Read the model definition and answer for the solid it produces. Units are mm, in the model's axes. A direction names the side the tool comes from. Give positions to 0.01 mm unless a question says otherwise; leave off trailing zeros. Order: outer loops, then holes, each group sorted by start corner. A loop starts at its lowest first (then second) coordinate and runs counter-clockwise, first axis right, second up. Notation, with made-up numbers: M 88,74 L 146,74 A29 ccw 146,100 Z; hole C 22.25,69.25 d5. An arc over 180 degrees is marked long. One line per item, written item: value.
from build123d import *

# Parameters (mm, degrees)
SKETCH1_W          = 50
SKETCH1_H          = 50
SKETCH1_R          = 7.875
BASE_FLANGE1_DEPTH = 1
FILLET1_R          = 3
FILLET2_R          = 1
FILLET3_R          = 2


# Sheet-metal steps are written as plain solids
with BuildPart() as part:
    # Sketch1 → Base-Flange1 (new body)
    with BuildSketch(Plane(origin=(0, 0, 0), x_dir=(1, 0, 0), z_dir=(0, 1, 0))):
        Rectangle(SKETCH1_W, SKETCH1_H)
        with Locations(Location((0, 0, 0), (0, 0, 270))):
            Circle(SKETCH1_R, mode=Mode.SUBTRACT)
        with BuildLine():
            Line((20, 17.878679656), (20, -17.878679656))
            Line((20, -17.878679656), (7.962313054, -5.84099271))
            ThreePointArc((7.962313054, -5.84099271), (9.875, 0), (7.962313054, 5.84099271))
            Line((7.962313054, 5.84099271), (20, 17.878679656))
        make_face(mode=Mode.SUBTRACT)
        with BuildLine():
            Line((17.878679656, -20), (-17.878679656, -20))
            Line((-17.878679656, -20), (-5.84099271, -7.962313054))
            ThreePointArc((-5.84099271, -7.962313054), (0, -9.875), (5.84099271, -7.962313054))
            Line((5.84099271, -7.962313054), (17.878679656, -20))
        make_face(mode=Mode.SUBTRACT)
        with BuildLine():
            Line((-20, -17.878679656), (-20, 17.878679656))
            Line((-20, 17.878679656), (-7.962313054, 5.84099271))
            ThreePointArc((-7.962313054, 5.84099271), (-9.875, 0), (-7.962313054, -5.84099271))
            Line((-7.962313054, -5.84099271), (-20, -17.878679656))
        make_face(mode=Mode.SUBTRACT)
        with BuildLine():
            Line((-17.878679656, 20), (17.878679656, 20))
            Line((17.878679656, 20), (5.84099271, 7.962313054))
            ThreePointArc((5.84099271, 7.962313054), (0, 9.875), (-5.84099271, 7.962313054))
            Line((-5.84099271, 7.962313054), (-17.878679656, 20))
        make_face(mode=Mode.SUBTRACT)
    extrude(amount=-BASE_FLANGE1_DEPTH)

    # Fillet1
    fillet1_edges = [part.edges().sort_by_distance(p)[0] for p in [
        (25, -0.5, 25),
        (-25, -0.5, 25),
        (-25, -0.5, -25),
        (25, -0.5, -25),
    ]]
    fillet(fillet1_edges, radius=FILLET1_R)

    # Fillet2
    fillet2_edges = [part.edges().sort_by_distance(p)[0] for p in [
        (17.878679656, -0.5, 20),
        (-17.878679656, -0.5, 20),
        (20, -0.5, -17.878679656),
        (20, -0.5, 17.878679656),
        (17.878679656, -0.5, -20),
        (-17.878679656, -0.5, -20),
        (-20, -0.5, -17.878679656),
        (-20, -0.5, 17.878679656),
    ]]
    fillet(fillet2_edges, radius=FILLET2_R)

    # Fillet3
    fillet3_edges = [part.edges().sort_by_distance(p)[0] for p in [
        (-5.84099271, -0.5, 7.962313054),
        (5.84099271, -0.5, 7.962313054),
        (7.962313054, -0.5, -5.84099271),
        (7.962313054, -0.5, 5.84099271),
        (5.84099271, -0.5, -7.962313054),
        (-5.84099271, -0.5, -7.962313054),
        (-7.962313054, -0.5, -5.84099271),
        (-7.962313054, -0.5, 5.84099271),
    ]]
    fillet(fillet3_edges, radius=FILLET3_R)


solid = part.part
1) Consider probe 1 along X at (y, z) = (-0.25, 0) (3 decimals); probe 2 along Z at (x, y) = (-5, -0.2); probe 3 along Z at (x, y) = (-19, -0.8). Determine where each line is inside the solid, lowest interval first.
Reported:
probe 1: x = -25 to -20, -9.875 to -7.875, 7.875 to 9.875, 20 to 25
probe 2: z = -25 to -20, -8.58 to -6.08, 6.08 to 8.58, 20 to 25
probe 3: z = -25 to -16.46, 16.46 to 25
2) Find section B-B, the plane x = 0. Write down the section's boundary in (y, z) (3 decimals).
Reported:
outline: M -1,-25 L 0,-25 L 0,-20 L -1,-20 Z; M -1,-9.875 L 0,-9.875 L 0,-7.875 L -1,-7.875 Z; M -1,7.875 L 0,7.875 L 0,9.875 L -1,9.875 Z; M -1,20 L 0,20 L 0,25 L -1,25 Z
3) This flat-tipped pin is pushed along its axis until it touches: pin 1 Ø14 at (x, z) = (0, 0) entering from -Y. Where does it stop, or does it pass through?
Reported:
pin 1: passes through
4) Find section A-A, the plane z = 0. Write down the section's boundary in (x, y) (3 decimals), plus the area to 3 significant figures.
Reported:
outline: M -25,-1 L -20,-1 L -20,0 L -25,0 Z; M -9.875,-1 L -7.875,-1 L -7.875,0 L -9.875,0 Z; M 7.875,-1 L 9.875,-1 L 9.875,0 L 7.875,0 Z; M 20,-1 L 25,-1 L 25,0 L 20,0 Z
area: 14.0 mm^2
5) Which of the six approach directions +Z, -Z, +X, -X, +Y, -Y give full straight-line access (tool end or side, diameter ignored) to faces 4 (the face through (-24.14, -0.51, 24.1)), 5 (the face through (13.75, -0.49, 11.63))?
Reported:
face 4: +Z, -X, +Y, -Y
face 5: +Y, -Y
6) Determine the mould class of faces 1 (the face through (-13.75, -0.49, -11.63)), 2 (the face through (-6, -1, -6)), 3 (the face through (24.1, -0.51, 24.14)) for opening direction X: +X half, -X half, draft (parallel to the pull), parting line (faces both ways), or undercut.
Reported:
face 1: undercut
face 2: draft
face 3: +X half
7) Find section C-C, the plane y = -0.6. Count the separate pieces of the cut face and the enclosed holes in it, plus the area to 3 significant figures.
Reported:
separate pieces: 1
enclosed holes: 5
area: 1,230 mm^2
